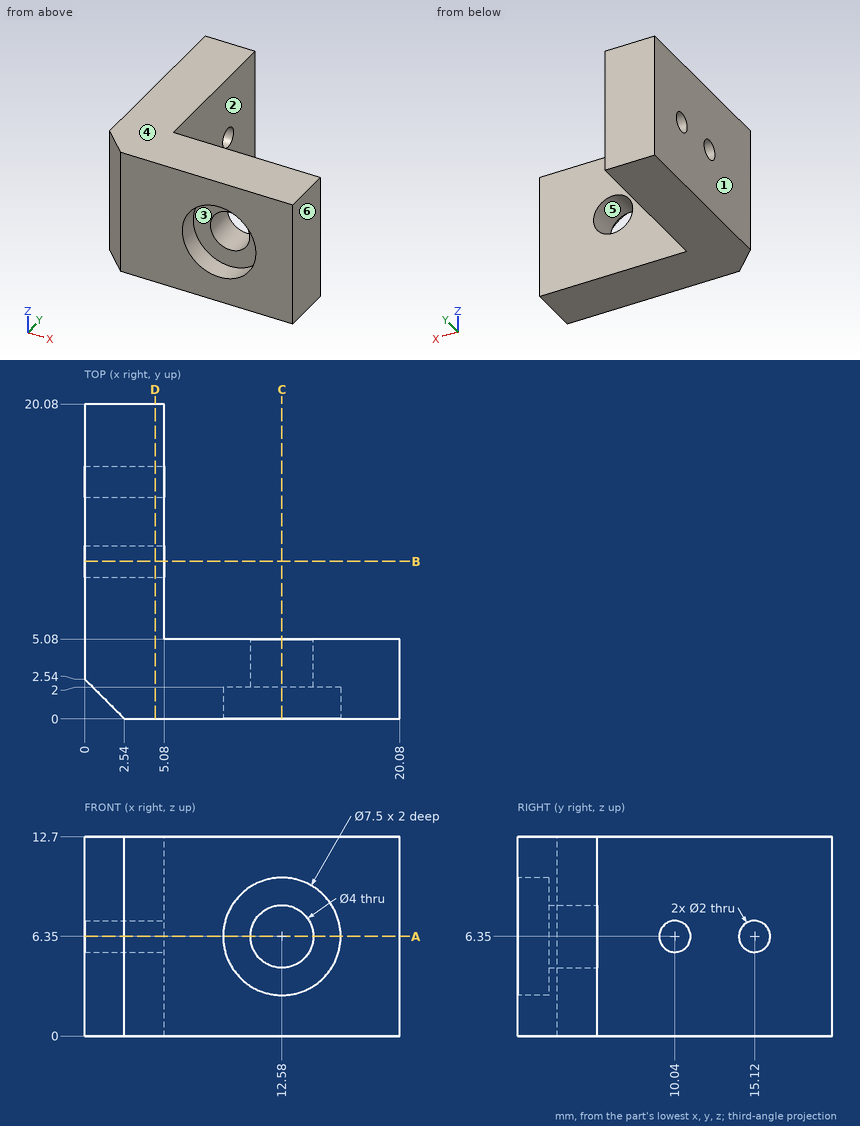
Study the drawing (mm; zero at the part's minimum x, y, z) and answer. A direction names the side the tool comes from. Coordinates: 2 decimals unless noted, no trailing zeros. Write each loop counter-clockwise with the first axis right and the second up, starting at its lowest first coordinate (ties: lowest second). Pieces come first, ordered by that corner, then holes. Notation, with made-up numbers: M -8.5,83 L 47.5,83 A7 ccw 47.5,88 Z; hole C -14.75,63.25 d11. An arc over 180 degrees is marked long. Use one line per item in the form item = value.
Item 1: Find section B-B, the plane y = 10.04. Give the vertices of the cut face in (x, z), plus the area to 3 significant figures.
Model answer:
outline = M 0,0 L 5.08,0 L 5.08,5.35 L 0,5.35 Z; M 0,7.35 L 5.08,7.35 L 5.08,12.7 L 0,12.7 Z
area = 54.4 mm2
Item 2: The mould has two halves that part along Z. Classify the marked faces 4, 5 and 6: released by +Z, released by -Z, zero draft, split by the parting line, or undercut.
Model answer:
face_4 = released by +Z
face_5 = undercut
face_6 = zero draft
Item 3: Find section D-D, the plane x = 4.5. Give the vertices of the cut face in (y, z).
Model answer:
outline = M 0,0 L 20.08,0 L 20.08,12.7 L 0,12.7 Z; hole C 10.04,6.35 d2; hole C 15.12,6.35 d2
Item 4: For the marked faces 1, 2 and 3, determine the directions among +Z, -Z, +X, -X, +Y, -Y from which every point of the face is accessible in a straight line to the end or side of a thin tool.
Model answer:
face_1 = +Z, -Z, -X, +Y, -Y
face_2 = +Z, -Z, +X, +Y
face_3 = -Y
Item 5: Find the intervals of material crossed by probe 1 along Z at (x, y) = (12.58, 1.3); probe 2 along Y at (x, z) = (1.75, 6.25); probe 3 along Z at (x, y) = (12.58, 2.7), in increasing order.
Model answer:
probe_1 = 0 to 2.6, 10.1 to 12.7
probe_2 = 0.79 to 9.05, 11.03 to 14.13, 16.11 to 20.08
probe_3 = 0 to 4.35, 8.35 to 12.7
Item 6: Given P1, Ø4, axis at x = 16, z = 4.5, coming from the +Y side; P2, Ø4.5, axis at x = 12.58, z = 6.35, coming from the -Y side; P3, Ø2.5, axis at y = 15.12, z = 6.35, coming from the +X side; P4, Ø6, axis at x = 5, y = 14.5, coming from the -Z side, each flat-ended and moving along its own axis, determine where each tip first touches the part or whether it passes through.
Model answer:
P1 = 5.08
P2 = 2
P3 = 5.08
P4 = 0
Item 7: Find section A-A, the plane z = 6.35. Give the vertices of the cut face in (x, y), plus the area to 3 significant figures.
Model answer:
outline = M 0,2.54 L 2.54,0 L 8.83,0 L 8.83,2 L 10.58,2 L 10.58,5.08 L 5.08,5.08 L 5.08,9.04 L 0,9.04 Z; M 0,11.04 L 5.08,11.04 L 5.08,14.12 L 0,14.12 Z; M 0,16.12 L 5.08,16.12 L 5.08,20.08 L 0,20.08 Z; M 14.58,2 L 16.33,2 L 16.33,0 L 20.08,0 L 20.08,5.08 L 14.58,5.08 Z
area = 127 mm2
Item 8: Find section C-C, the plane x = 12.58. Give the vertices of the cut face in (y, z), plus the area to 3 significant figures.
Model answer:
outline = M 0,0 L 5.08,0 L 5.08,4.35 L 2,4.35 L 2,2.6 L 0,2.6 Z; M 0,10.1 L 2,10.1 L 2,8.35 L 5.08,8.35 L 5.08,12.7 L 0,12.7 Z
area = 37.2 mm2
